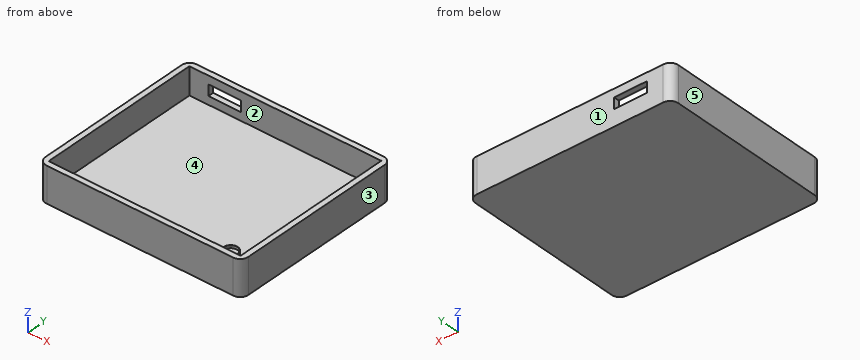
Autodesk Fusion 360 part; units mm, degrees
sketch "Sketch3" plane through (0, 0, 0) normal (0, 0, 1) x (1, 0, 0)
  line L0 (0, 0) -> (74.4, 0)
  line L1 (74.4, 0) -> (74.4, -64.4)
  line L2 (74.4, -64.4) -> (0, -64.4)
  line L3 (0, -64.4) -> (0, 0)
  dimension "d8" = 74.4
  dimension "d9" = 64.4
extrude "Extrude2" add sketch "Sketch3" along normal blind 3
sketch "Sketch4" plane through (0, 0, 3) normal (0, 0, 1) x (-1, 0, 0)
  line L0 (0, 64.4) -> (-74.4, 64.4)
  line L1 (-74.4, 64.4) -> (-74.4, 0)
  line L2 (-74.4, 0) -> (0, 0)
  line L3 (0, 0) -> (0, 64.4)
  line L4 (0, 0) -> (-74.4, 0)
  line L5 (-74.4, 0) -> (-74.4, 2)
  line L6 (-74.4, 2) -> (0, 2)
  line L7 (0, 2) -> (0, 0)
  line L8 (-74.4, 0) -> (-72.4, 0)
  line L9 (-72.4, 0) -> (-72.4, 64.4)
  line L10 (-72.4, 64.4) -> (-74.4, 64.4)
  line L11 (-74.4, 64.4) -> (-74.4, 0)
  line L12 (0, 0) -> (-2, 0)
  line L13 (-2, 0) -> (-2, 64.4)
  line L14 (-2, 64.4) -> (0, 64.4)
  line L15 (0, 64.4) -> (0, 0)
  line L16 (0, 64.4) -> (-74.4, 64.4)
  line L17 (-74.4, 64.4) -> (-74.4, 62.4)
  line L18 (-74.4, 62.4) -> (0, 62.4)
  line L19 (0, 62.4) -> (0, 64.4)
  dimension "d12" = 2
  dimension "d13" = 2
  dimension "d14" = 2
  dimension "d15" = 2
extrude "Extrude3" add sketch "Sketch4" along normal blind 10 contours L0 L3 L13 L14 L15 L16 L18 L19 | L0 L9 L13 L16 L18 | L3 L6 L13 L15 L18 | L0 L1 L9 L10 L11 L16 L17 L18 | L2 L3 L4 L6 L7 L12 L13 L15 | L1 L6 L9 L11 L18 | L2 L4 L6 L9 L13 | L1 L2 L4 L5 L6 L8 L9 L11
sketch "Sketch6" plane through (0, 0, 0) normal (0, 1, 0) x (-1, 0, 0)
  line L0 (-74.4, 0) -> (0, 0)
  line L1 (0, 0) -> (0, 13)
  line L2 (0, 13) -> (-74.4, 13)
  line L3 (-74.4, 13) -> (-74.4, 0)
  line L4 (-8.3, 5) -> (-22.3, 5)
  line L5 (-22.3, 5) -> (-22.3, 9)
  line L6 (-22.3, 9) -> (-8.3, 9)
  line L7 (-8.3, 9) -> (-8.3, 5)
  dimension "d23" = 14
  dimension "d24" = 8.3
  dimension "d25" = 5
fillet "Fillet1" radius 3 4 edges at (74.4, -64.4, 6.5) (74.4, 0, 6.5) (0, 0, 6.5) (0, -64.4, 6.5)
sketch "Sketch7" plane through (0, 0, 3) normal (0, 0, 1) x (-1, 0, 0)
  line L0 (-2, 62.4) -> (-72.4, 62.4)
  line L1 (-72.4, 62.4) -> (-72.4, 2)
  line L2 (-72.4, 2) -> (-2, 2)
  line L3 (-2, 2) -> (-2, 62.4)
  circle A0 centre (-62.2, 54.7) radius 2.6
  dimension "d30" = 5.2
  dimension "d31" = 10.2
  dimension "d32" = 7.7
extrude "Extrude5" add sketch "Sketch7" along normal blind 3 contours A0
sketch "Sketch8" plane through (0, 0, 6) normal (0, 0, 1) x (-1, 0, 0)
  circle A0 centre (-62.2, 54.7) radius 2.6
  circle A1 centre (-62.2, 54.7) radius 2.5
  dimension "d35" = 5
extrude "Extrude6" cut sketch "Sketch8" against normal blind 1 contours A1
sketch "Sketch10" plane through (0, -2, 0) normal (0, -1, 0) x (1, 0, 0)
  line L0 (2, 3) -> (72.4, 3)
  line L1 (72.4, 3) -> (72.4, 13)
  line L2 (72.4, 13) -> (2, 13)
  line L3 (2, 13) -> (2, 3)
  line L4 (9, 6) -> (21, 6)
  line L5 (21, 6) -> (21, 10)
  line L6 (21, 10) -> (9, 10)
  line L7 (9, 10) -> (9, 6)
  dimension "d46" = 12
  dimension "d47" = 4
  dimension "d48" = 3
  dimension "d49" = 7
extrude "Extrude8" cut sketch "Sketch10" against normal blind 3 contours L4 L5 L6 L7
Geometry check sheet. Reference: the model listing, model coordinates, mm. Face numbers are marked on the shaded views. A direction names the side the tool comes from. Coordinates: 2 decimals unless noted, no trailing zeros. Order: outer loops, then holes, each group sorted by start corner. A loop starts at its lowest first (then second) coordinate and runs counter-clockwise, first axis right, second up. Notation, with made-up numbers: M 10.25,53.5 L 26.25,53.5 A26 cw 26.25,92.5 Z; hole C 65.5,87.5 d10. An arc over 180 degrees is marked long. Answer as a JSON object with one key per item and string values.
Q1. Cross-section at B-B on y = -54.7. Record the cut outline in (x, z).
Results are:
{"outline": "M 0,0 L 74.4,0 L 74.4,13 L 72.4,13 L 72.4,3 L 64.8,3 L 64.8,6 L 64.7,6 L 64.7,5 L 59.7,5 L 59.7,6 L 59.6,6 L 59.6,3 L 2,3 L 2,13 L 0,13 Z"}
Q2. Cross-section at A-A on z = 4. Record the cut outline in (x, y).
Results are:
{"outline": "M 0,-61.4 A3 ccw 3,-64.4 L 71.4,-64.4 A3 ccw 74.4,-61.4 L 74.4,-3 A3 ccw 71.4,0 L 3,0 A3 ccw 0,-3 Z; C 62.2,-54.7 d5.2; hole M 2,-62.4 L 72.4,-62.4 L 72.4,-2 L 2,-2 Z"}
Q3. Cross-section at C-C on z = 11.75. Record the cut outline in (x, y).
Results are:
{"outline": "M 0,-61.4 A3 ccw 3,-64.4 L 71.4,-64.4 A3 ccw 74.4,-61.4 L 74.4,-3 A3 ccw 71.4,0 L 3,0 A3 ccw 0,-3 Z; hole M 2,-62.4 L 72.4,-62.4 L 72.4,-2 L 2,-2 Z"}
Q4. Cross-section at D-D on x = 62.2. Record the cut outline in (y, z).
Results are:
{"outline": "M -64.4,0 L 0,0 L 0,13 L -2,13 L -2,3 L -52.1,3 L -52.1,6 L -52.2,6 L -52.2,5 L -57.2,5 L -57.2,6 L -57.3,6 L -57.3,3 L -62.4,3 L -62.4,13 L -64.4,13 Z"}
Q5. Depth check by flat-ended pin: pin 1 Ø3 at (x, z) = (33.5, 10.5) entering from +Y; pin 2 Ø2 at (y, z) = (-1.5, 8) entering from +X; pin 3 Ø2.5 at (x, y) = (62, -55) entering from +Z; pin 4 Ø2 at (y, z) = (-1, 9) entering from -X. Enter the tip coordinate at first touch or a pass-through.
Results are:
{"pin 1": "stops at y = 0", "pin 2": "stops at x = 74.36", "pin 3": "stops at z = 5", "pin 4": "stops at x = 0.17"}
Q6. Scan lines: line 1 (X direction, y = -20.5, z = 3.5); line 2 (Y direction, x = 3, z = 3.75); line 3 (Z direction, x = 6.5, y = -33.5). Record each from-to range of solid material in increasing order.
Results are:
{"line 1": "x = 0 to 2, 72.4 to 74.4", "line 2": "y = -64.4 to -62.4, -2 to 0", "line 3": "z = 0 to 3"}
Q7. Release check for a two-part mould opening along X. For the marked faces 1, 2 and 3 record: released by +X, released by -X, zero draft, split by the parting line, or undercut.
Results are:
{"face 1": "zero draft", "face 2": "undercut", "face 3": "released by +X"}
Q8. Tool access check on the marked faces 4 and 5. Record the directions out of +Z, -Z, +X, -X, +Y, -Y that give a thin tool (end or side, any length) a straight path to the whole face; none if there is none.
Results are:
{"face 4": "+Z", "face 5": "+Z, -Z, -X, +Y, -Y"}
